Solid Edge part; units mm, degrees
sketch "Sketch1" plane through (0, 0, 0) normal (0, -1, 0) x (1, 0, 0)
  circle A0 centre (0, 0) radius 21
extrude "Extrusionsausprägung_1" add sketch "Sketch1" along normal blind 3
sketch "Sketch2" plane through (0, -3, 0) normal (0, -1, 0) x (1, 0, 0)
  circle A0 centre (0, 0) radius 18.25
extrude "Extrusionsausprägung_2" add sketch "Sketch2" along normal blind 8
sketch "Sketch3" plane through (0, -11, 0) normal (0, -1, 0) x (1, 0, 0)
  circle A0 centre (0, 0) radius 9.75
extrude "Extrusionsausprägung_3" add sketch "Sketch3" along normal blind 4.2
sketch "Sketch4" plane through (0, -15.2, 0) normal (0, -1, 0) x (1, 0, 0)
  circle A0 centre (0, 0) radius 18.25
extrude "Extrusionsausprägung_4" add sketch "Sketch4" along normal blind 6
fillet "Verrundung_1" radius 1.5 1 edges at (-18.25, -21.2, 0)
hole "Bohrung_1" at (0, -21.2, 0) direction (0, 1, 0) diameter 6 end through all
properties material "ABS-Plastik, mittlerer Anschlag"
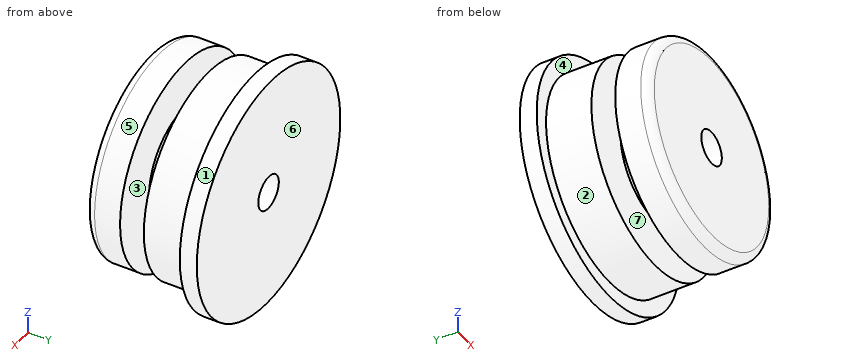
Geometry: final body of the model. Coordinates: model frame, mm. Face numbers are marked on the shaded views. A direction names the side the tool comes from. Give positions to 0.01 mm unless a question says otherwise; leave off trailing zeros. Loops run counter-clockwise (first coordinate to the right, second up) from the corner with the lowest first, then second, coordinate; pieces in that order, holes last. Notation, with made-up numbers: (53, -10.75) - (111, -10.75) arc R26 cw to (111, 10.25) - close; hole circle Ø6 at (-27.5, 88.5). An arc over 180 degrees is marked (long way). Answer as CSV lines item,"result". Start each with the question number.
1. Draft query along Y for the marked faces 4, 5, 6 and 7. Return one class per face: released by +Y, released by -Y, zero draft, split by the parting line, or undercut.
2. Reachability of the marked faces 1, 2 and 3 from +Z, -Z, +X, -X, +Y, -Y: full face, straight path, thin tool, end or side. Return the list, or none.
3. Ray query, L1, parallel to Y at x = 14.5, z = -7; L2, parallel to Z at x = 0, y = -11.75; L3, parallel to Z at x = 0, y = -6.25. Return the intervals inside material, ascending.
4. Section D-D, the plane y = -11.75. Return loops of the section in (x, z).
5. Pin query (flat end, axial travel): P1, Ø10, axis at x = -15, y = -3, coming from the +Z side; P2, Ø1, axis at x = 5, z = -7, coming from the +Y side; P3, Ø8, axis at y = -8, z = -10, coming from the +X side; P4, Ø1.5, axis at y = -4.5, z = -6.5, coming from the +X side. Return the tip coordinate at first contact, or that it passes through.
6. Section C-C, the plane y = -7.5. Return loops of the section in (x, z), plus the area to 3 significant figures.
7. Section A-A, the plane z = 0. Return loops of the section in (x, y), plus the area to 3 significant figures.
8. Section B-B, the plane x = 0. Return loops of the section in (y, z).
Answers:
1,face 4,"released by -Y"
1,face 5,"zero draft"
1,face 6,"released by +Y"
1,face 7,"undercut"
2,face 1,"+Y, -Y"
2,face 2,"-Y"
2,face 3,"none"
3,L1,"y = -21.2 to -15.2, -11 to 0"
3,L2,"z = -9.75 to -3, 3 to 9.75"
3,L3,"z = -18.25 to -3, 3 to 18.25"
4,outline,"circle Ø19.5 at (0, 0); hole circle Ø6 at (0, 0)"
5,P1,"stops at z = 18.47"
5,P2,"stops at y = 0"
5,P3,"stops at x = 17.24"
5,P4,"stops at x = 17.32"
6,outline,"circle Ø36.5 at (0, 0); hole circle Ø6 at (0, 0)"
6,area,"1,020 mm2"
7,outline,"(-21, -3) - (-18.25, -3) - (-18.25, -11) - (-9.75, -11) - (-9.75, -15.2) - (-18.25, -15.2) - (-18.25, -19.7) arc R1.5 ccw to (-16.75, -21.2) - (-3, -21.2) - (-3, 0) - (-21, 0) - close; (3, -21.2) - (16.75, -21.2) arc R1.5 ccw to (18.25, -19.7) - (18.25, -15.2) - (9.75, -15.2) - (9.75, -11) - (18.25, -11) - (18.25, -3) - (21, -3) - (21, 0) - (3, 0) - close"
7,area,"591 mm2"
8,outline,"(-21.2, -16.75) arc R1.5 ccw to (-19.7, -18.25) - (-15.2, -18.25) - (-15.2, -9.75) - (-11, -9.75) - (-11, -18.25) - (-3, -18.25) - (-3, -21) - (0, -21) - (0, -3) - (-21.2, -3) - close; (-21.2, 3) - (0, 3) - (0, 21) - (-3, 21) - (-3, 18.25) - (-11, 18.25) - (-11, 9.75) - (-15.2, 9.75) - (-15.2, 18.25) - (-19.7, 18.25) arc R1.5 ccw to (-21.2, 16.75) - close"
